```python
from build123d import *

# Parameters (mm, degrees)
SKETCH001_R  = 1
PAD_DEPTH    = 5
SKETCH002_R  = 0.5
POCKET_DEPTH = 10


with BuildPart() as part:
    # Sketch001 → Pad (new body)
    with BuildSketch(Plane.XY):
        Polygon((9, 0), (9, 15), (0, 15), (0, 40), (50, 40), (50, 15), (41, 15), (41, 0), (31, 0), (31, 25), (19, 25), (19, 0), align=None)
        with Locations((46.504002, 36.501442)):
            Circle(SKETCH001_R, mode=Mode.SUBTRACT)
        with Locations((3.500559, 36.501442)):
            Circle(SKETCH001_R, mode=Mode.SUBTRACT)
        with Locations((3.500559, 18.503159)):
            Circle(SKETCH001_R, mode=Mode.SUBTRACT)
        with Locations((46.496666, 18.503159)):
            Circle(SKETCH001_R, mode=Mode.SUBTRACT)
    extrude(amount=PAD_DEPTH)

    # Sketch002 (on Face9 of Pad) → Pocket (cut)
    with BuildSketch(Plane.XZ):
        with Locations((38.496052, 2.503616)):
            Circle(SKETCH002_R)
        with Locations((33.499767, 2.503616)):
            Circle(SKETCH002_R)
        with Locations((16.502573, 2.498577)):
            Circle(SKETCH002_R)
        with Locations((11.496223, 2.503616)):
            Circle(SKETCH002_R)
    extrude(amount=-POCKET_DEPTH, mode=Mode.SUBTRACT)


solid = part.part
```
Check sheet for the modelled part. Datum: model origin and axes. Units: mm. A direction names the side the tool comes from. Round coordinates to 2 decimals unless told otherwise and drop trailing zeros. Loops run counter-clockwise (first coordinate to the right, second up) from the corner with the lowest first, then second, coordinate; pieces in that order, holes last. Notation, with made-up numbers: (19, 31) -> (58, 31) arc R10 ccw to (58, 43) -> close; hole circle Ø2 at (-11, -7.5). An arc over 180 degrees is marked (long way). Write item = value, one per line. Start each with the question number.
1) Sectioned sample at C-C, the plane x = 22. Record the cut outline in (y, z), plus the area to 3 significant figures.
2) Release check for a two-part mould opening along Z. For faces 1 (the flat face through (25, 25, 2)), 2 (the flat face through (38.5, 10, 2.5)), 3 (the flat face through (25, 29, 0)) record: released by +Z, released by -Z, zero draft, split by the parting line, or undercut.
3) Sectioned sample at A-A, the plane y = 21. Record the cut outline in (x, z).
4) Sectioned sample at B-B, the plane z = 0.6. Record the cut outline in (x, y), plus the area to 3 significant figures.
5) Gauge pin test, flat ends, axial feed: pin 1 Ø0.5 at (x, z) = (38.5, 2.5) entering from -Y; pin 2 Ø3 at (x, y) = (3.5, 18.5) entering from -Z; pin 3 Ø1.5 at (y, z) = (8.5, 1.5) entering from -X; pin 4 Ø1.5 at (x, z) = (27.5, 2) entering from -Y. Record the tip position at first contact, or that the pin passes through.
6) Set-up check for faces 4 (the flat face through (33.5, 10, 2.5)), 5 (the flat face through (19, 13, 2)), 6 (the flat face through (5, 15, 2)), 7 (the flat face through (46, 15, 2)): record each of +Z, -Z, +X, -X, +Y, -Y from which the full face is reachable in a straight line by a thin tool's end or side.
7) Thickness scan on probe 1 along Y at (x, z) = (46.5, 1.6); probe 2 along X at (y, z) = (13, 0.55); probe 3 along X at (y, z) = (22, 1.8). Record the ranges inside material, lowest first.
Results are:
q1.outline = (25, 0) -> (40, 0) -> (40, 5) -> (25, 5) -> close
q1.area = 75.0 mm^2
q2.face_1 = zero draft
q2.face_2 = undercut
q2.face_3 = released by -Z
q3.outline = (0, 0) -> (19, 0) -> (19, 5) -> (0, 5) -> close; (31, 0) -> (50, 0) -> (50, 5) -> (31, 5) -> close
q4.outline = (0, 15) -> (9, 15) -> (9, 0) -> (19, 0) -> (19, 25) -> (31, 25) -> (31, 0) -> (41, 0) -> (41, 15) -> (50, 15) -> (50, 40) -> (0, 40) -> close; hole circle Ø2 at (3.5, 18.5); hole circle Ø2 at (3.5, 36.5); hole circle Ø2 at (46.5, 18.5); hole circle Ø2 at (46.5, 36.5)
q4.area = 1,420 mm^2
q5.pin_1 = 10
q5.pin_2 = 0
q5.pin_3 = 9
q5.pin_4 = 25
q6.face_4 = -Y
q6.face_5 = +Z, -Z, -Y
q6.face_6 = +Z, -Z, -X, -Y
q6.face_7 = +Z, -Z, +X, -Y
q7.probe_1 = 15 to 17.5, 19.5 to 35.5, 37.5 to 40
q7.probe_2 = 9 to 19, 31 to 41
q7.probe_3 = 0 to 19, 31 to 50
